```python
from build123d import *

# Parameters (mm, degrees)
F0_W     = 60
F0_H     = 43.5
F0_R     = 3.075
F1_DEPTH = 20
F0_R_2   = 1
F2_DEPTH = 27
F3_W     = 60
F3_H     = 8.5
F4_DEPTH = 10
F5_R     = 5
F6_SIZE  = 1


with BuildPart() as f1:
    # F0 (on Top) → F1 (new body)
    with BuildSketch(Plane.XY):
        with Locations((30, 21.75)):
            Rectangle(F0_W, F0_H)
        with Locations((10, 10)):
            Circle(F0_R, mode=Mode.SUBTRACT)
        with Locations((50, 10)):
            Circle(F0_R, mode=Mode.SUBTRACT)
        with Locations((10, 25)):
            Circle(F0_R, mode=Mode.SUBTRACT)
        with Locations((50, 25)):
            Circle(F0_R, mode=Mode.SUBTRACT)
    extrude(amount=F1_DEPTH)

    # F0 (on Top) → F2 (join)
    with BuildSketch(Plane.XY):
        with Locations((10, 25)):
            Circle(F0_R)
        with Locations((10, 25)):
            Circle(F0_R_2, mode=Mode.SUBTRACT)
        with Locations((10, 10)):
            Circle(F0_R)
        with Locations((10, 10)):
            Circle(F0_R_2, mode=Mode.SUBTRACT)
        with Locations((50, 10)):
            Circle(F0_R)
        with Locations((50, 10)):
            Circle(F0_R_2, mode=Mode.SUBTRACT)
        with Locations((50, 25)):
            Circle(F0_R)
        with Locations((50, 25)):
            Circle(F0_R_2, mode=Mode.SUBTRACT)
    extrude(amount=F2_DEPTH)

    # F3 (on face) → F4 (cut)
    with BuildSketch(Plane.XY.offset(20)):
        with Locations((30, 39.25)):
            Rectangle(F3_W, F3_H)
    extrude(amount=-F4_DEPTH, mode=Mode.SUBTRACT)

    # F5
    f5_edges = [f1.edges().sort_by_distance(p)[0] for p in [
        (60, 0, 10),
        (0, 0, 10),
        (60, 43.5, 5),
        (60, 35, 15),
        (0, 35, 15),
        (0, 43.5, 5),
    ]]
    fillet(f5_edges, radius=F5_R)

    # F6
    f6_edges = [f1.edges().sort_by_distance(p)[0] for p in [
        (30, 35, 20),
        (1.464466, 33.535534, 20),
        (58.535534, 33.535534, 20),
        (0, 17.5, 20),
        (60, 17.5, 20),
        (1.464466, 1.464466, 20),
        (58.535534, 1.464466, 20),
        (30, 0, 20),
        (6.925, 10, 20),
        (46.925, 10, 20),
        (6.925, 25, 20),
        (46.925, 25, 20),
        (6.925, 10, 27),
        (6.925, 25, 27),
        (46.925, 25, 27),
        (46.925, 10, 27),
        (30, 43.5, 10),
        (58.535534, 42.035534, 10),
    ]]
    chamfer(f6_edges, length=F6_SIZE)


solid = f1.part
```
Here's how the part is built. I have some questions about the finished solid (model axes, mm). A direction names the side the tool comes from. Give positions to 0.01 mm unless a question says otherwise; leave off trailing zeros. Write each loop counter-clockwise with the first axis right and the second up, starting at its lowest first coordinate (ties: lowest second). Pieces come first, ordered by that corner, then holes. Notation, with made-up numbers: (30.5, 62) -> (40.5, 62) arc R24 ccw to (40.5, 94) -> close; hole circle Ø6 at (-23.5, -40). An arc over 180 degrees is marked (long way). Write each question's results on one line, items separated by ' | '.
Item 1: If I drill on L1, parallel to Y at x = 50, z = 7.5; L2, parallel to Y at x = 50, z = 13.25; L3, parallel to X at y = 24.5, z = 10, over which ranges is the centre line in solid material (lowest first)?
Output:
L1: y = 0 to 9, 11 to 24, 26 to 43.5 | L2: y = 0 to 9, 11 to 24, 26 to 35 | L3: x = 0 to 9.13, 10.87 to 49.13, 50.87 to 60
Item 2: Suppose I cut it at C-C on x = 22. Write out the boundary of the cut face in (y, z).
Output:
outline: (0, 0) -> (43.5, 0) -> (43.5, 9) -> (42.5, 10) -> (35, 10) -> (35, 19) -> (34, 20) -> (1, 20) -> (0, 19) -> close
Item 3: Suppose I cut it at A-A on y = 25. Give the number of separate pieces and of enclosed holes in the cut face, plus the area to 3 significant figures.
Output:
separate pieces: 3 | enclosed holes: 0 | area: 1,180 mm^2
Item 4: We'd pull the mould along X, two halves only. Please class faces 4 (the face through (59, 2, 10)), 5 (the face through (30, 22, 0)), 6 (the face through (0, 22, 9)), 7 (the face through (51, 10, 13)): pulls with the +X half, pulls with the -X half, needs draft (parallel to the pull), parting line crosses it, or undercut.
Output:
face 4: pulls with the +X half | face 5: needs draft | face 6: pulls with the -X half | face 7: undercut
Item 5: For pin 1 Ø1.2 at (x, y) = (10, 25) entering from +Z; pin 2 Ø3 at (x, y) = (18.5, 11) entering from +Z; pin 3 Ø2.5 at (x, z) = (35, 14) entering from +Y; pin 4 Ø4 at (y, z) = (30, 21.5) entering from +X, each with a flat end and sliding along its axis, tell me the tip position at first contact or that it passes through.
Output:
pin 1: passes through | pin 2: stops at z = 20 | pin 3: stops at y = 35 | pin 4: stops at x = 59.5
Item 6: Suppose I cut it at D-D on y = 20. Write out the boundary of the cut face in (x, z).
Output:
outline: (0, 0) -> (60, 0) -> (60, 19) -> (59, 20) -> (1, 20) -> (0, 19) -> close
Item 7: On a 3-axis mill with a long thin cutter (end or side, diameter ignored), from which of +Z, -Z, +X, -X, +Y, -Y can I reach the whole of each face in a straight line? I mean faces 1 (the face through (58, 34, 14)), 2 (the face through (58.063, 2.004, 19.715)), 3 (the face through (7.734, 12.078, 23.465)). Say none if no direction works.
Output:
face 1: +Z, +X, +Y | face 2: +Z, +X, -Y | face 3: +Z
